Can you work these out from the model? Positions are in its coordinate system, mm. A direction names the side the tool comes from. Round coordinates to 2 decimals unless told otherwise and drop trailing zeros. Order: outer loops, then holes, each group sorted by start corner. A loop starts at its lowest first (then second) coordinate and runs counter-clockwise, first axis right, second up. Notation, with made-up numbers: (-20.5, -21) -> (20.5, -21) arc R17 ccw to (20.5, 4) -> close; hole circle Ø11 at (54.25, 13). An arc over 180 degrees is marked (long way). Use a Markdown table: item, result. Add a question column.
Q1. If we section it at A-A on z = -340.1: List the corners of the cut face in (x, y) for me.
Q2. I need wall thicknesses on line 1 along Z through (x, y) = (-13.95, 1.5); line 2 along X through (y, z) = (1.25, -370); line 3 along Y through (x, z) = (-13.55, -505.2). Which ranges of each line are inside material? Lowest first, please. Write a range as [from, to].
Q3. If we section it at B-B on y = 1.5: List the corners of the cut face in (x, z) for me, plus the area to 3 significant figures.
Q4. I'm going to push flat-ended pins straight in: pin 1 Ø10 at (x, z) = (3.5, -359) entering from +Y; pin 2 Ø9.5 at (y, z) = (1.5, -340.1) entering from -X. Where does each tip first touch, or does it pass through?
Q5. If we section it at C-C on z = -180.5: List the corners of the cut face in (x, y) for me.
Q6. For faces 1 (the face through (-16, 0, -275)), 2 (the face through (-14.521, 1.236, -334.106)), 3 (the face through (-13, 2, -275)), which set-ups out of +Z, -Z, +X, -X, +Y, -Y let a thin tool reach every point of the face, with its end or its side?
Q7. We'd pull the mould along Z, two halves only. Please class faces 4 (the face through (0, -9.5, -275)), 5 (the face through (-14.521, -0.302, -420.923)), 6 (the face through (-1, -10, -558.8)), 7 (the face through (-14.521, 1.236, -244.106)): +Z half, -Z half, draft (parallel to the pull), parting line (faces both ways), or undercut.
Autodesk Inventor part; units mm, degrees
ref_plane "YZ Plane" through (0, 0, 0) normal (1, 0, 0) x (0, 1, 0)
ref_plane "XZ Plane" through (0, 0, 0) normal (0, 1, 0) x (-1, 0, 0)
ref_plane "XY Plane" through (0, 0, 0) normal (0, 0, 1) x (1, 0, 0)
sketch "Sketch1" plane through (0, 0, 0) normal (0, 0, 1) x (1, 0, 0)
  line L0 (-16, 12.5) -> (-13, 12.5)
  line L1 (-13, 12.5) -> (-13, -9.5)
  line L2 (-13, -9.5) -> (13, -9.5)
  line L3 (13, -9.5) -> (13, 12.5)
  line L4 (13, 12.5) -> (16, 12.5)
  line L5 (16, 12.5) -> (16, -12.5)
  line L6 (16, -12.5) -> (-16, -12.5)
  line L7 (-16, -12.5) -> (-16, 12.5)
  point P0 (0, 0)
  dimension "d0" = 3
  dimension "d2" = 3
  dimension "d3" = 25
  dimension "d4" = 32
  dimension "d5" = 16
  dimension "d7" = 12.5
  dimension "d8" = 3
  dimension "d74" = 25
extrude "Extrusion1" add sketch "Sketch1" against normal blind 558.8
sketch "Sketch8" plane through (-16, -12.5, 0) normal (0, -1, 0) x (1, 0, 0)
  line L0 (32, -558.8) -> (0, -558.8)
  line L1 (32, 0) -> (32, -558.8)
  circle A0 centre (16, -547.8) radius 3.175
  line L2 (32, 0) -> (0, 0)
  circle A1 centre (16, -11) radius 3.175
  point P0 (16, 0)
  dimension "d114" = 6.35
  dimension "d116" = 16
  dimension "d117" = 11
  dimension "d125" = 6.35
  dimension "d126" = 11
hole "Hole5" at (0, -12.5, -547.8) at (0, -12.5, -11) direction (0, 1, 0) diameter 6.35 end through all
sketch "Sketch9" plane through (-13, -9.5, 0) normal (1, 0, 0) x (0, 0, -1)
  circle A0 centre (505.2, 11) radius 6
  circle A1 centre (415.2, 11) radius 6
  circle A2 centre (340.1, 11) radius 6
  circle A3 centre (250.1, 11) radius 6
  point P0 (0, 9.5)
hole "Hole6" at (-13, 1.5, -340.1) at (-13, 1.5, -250.1) at (-13, 1.5, -505.2) at (-13, 1.5, -415.2) direction (-1, 0, 0) diameter 12 depth 3 tip angle 118
equation "\"d2\" = d0"
equation "\"d8\" = d0"
equation "\"d74\" = d3"
equation "\"d126\" = d117"
properties part number "Shooter Frame - CIM Mount" material "Aluminum 6061"
Answer below:
| question | item | result |
|---|---|---|
| 1 | outline | (-16, -12.5) -> (16, -12.5) -> (16, 12.5) -> (13, 12.5) -> (13, -9.5) -> (-13, -9.5) -> (-13, -4.5) -> (-16, -4.5) -> close; (-16, 7.5) -> (-13, 7.5) -> (-13, 12.5) -> (-16, 12.5) -> close |
| 2 | line 1 | [-558.8, -511.2], [-499.2, -421.2], [-409.2, -346.1], [-334.1, -256.1], [-244.1, 0] |
| 2 | line 2 | [-16, -13], [13, 16] |
| 2 | line 3 | [-12.5, -4.5], [7.5, 12.5] |
| 3 | outline | (-16, -558.8) -> (-13, -558.8) -> (-13, -511.2) -> (-16, -511.2) -> close; (-16, -499.2) -> (-13, -499.2) -> (-13, -421.2) -> (-16, -421.2) -> close; (-16, -409.2) -> (-13, -409.2) -> (-13, -346.1) -> (-16, -346.1) -> close; (-16, -334.1) -> (-13, -334.1) -> (-13, -256.1) -> (-16, -256.1) -> close; (-16, -244.1) -> (-13, -244.1) -> (-13, 0) -> (-16, 0) -> close; (13, -558.8) -> (16, -558.8) -> (16, 0) -> (13, 0) -> close |
| 3 | area | 3,210 mm² |
| 4 | pin 1 | y = -9.5 |
| 4 | pin 2 | x = 13 |
| 5 | outline | (-16, -12.5) -> (16, -12.5) -> (16, 12.5) -> (13, 12.5) -> (13, -9.5) -> (-13, -9.5) -> (-13, 12.5) -> (-16, 12.5) -> close |
| 6 | face 1 | +Z, -Z, -X, +Y, -Y |
| 6 | face 2 | -X |
| 6 | face 3 | +Z, -Z, +Y |
| 7 | face 4 | draft |
| 7 | face 5 | undercut |
| 7 | face 6 | -Z half |
| 7 | face 7 | undercut |
